from build123d import *

# Parameters (mm, degrees)
F0_R     = 1.95
F1_DEPTH = 30
F2_SIZE  = 1
F0_W     = 62.6598149538
F0_H     = 31.0992728919
F0_R_2   = 15
F3_DEPTH = 3
F4_D     = 3.3
F4_DEPTH = 10
F4_TIP   = 0.9914200214


with BuildPart() as f1:
    # F0 (on Top) → F1 (new body)
    with BuildSketch(Plane.XY):
        Circle(F0_R)
    extrude(amount=F1_DEPTH)

    # F2
    f2_edges = [f1.edges().sort_by_distance(p)[0] for p in [
        (-1.95, 0, 30),
    ]]
    chamfer(f2_edges, length=F2_SIZE)

    # F0 (on Top) → F3 (join)
    with BuildSketch(Plane.XY):
        Rectangle(F0_W, F0_H)
        Circle(F0_R_2, mode=Mode.SUBTRACT)
        Circle(F0_R_2)
        Circle(F0_R, mode=Mode.SUBTRACT)
        Circle(F0_R)
    extrude(amount=-F3_DEPTH)

    # F4
    with Locations(Plane.XY):
        with Locations((-26.3299074769, 10.5496364459), (26.3299074769, 10.5496364459), (26.3299074769, -10.5496364459), (-26.3299074769, -10.5496364459)):
            Hole(F4_D / 2, depth=F4_DEPTH)
            with Locations((0, 0, -(F4_DEPTH + F4_TIP / 2))):  # 118° drill point
                Cone(0, F4_D / 2, F4_TIP, mode=Mode.SUBTRACT)


solid = f1.part
Input: part model. Units: mm. Frame: model coordinates. Give positions to 0.01 mm unless a question says otherwise; leave off trailing zeros. Write each loop counter-clockwise with the first axis right and the second up, starting at its lowest first coordinate (ties: lowest second). Pieces come first, ordered by that corner, then holes.
Q1. First-contact query: P1, Ø3, axis at x = 5, z = 15.5, coming from the -Y side; P2, Ø8, axis at x = 4, y = -4, coming from the +Z side; P3, Ø4.5, axis at x = -26.33, y = 10.55, coming from the +Z side. Flat tips, straight axial feed; report the tip coordinate or a pass-through.
Q2. Section D-D, the plane x = 20. Output: boundary loops of the cut face in (y, z), plus the area to 3 significant figures.
Q3. Section C-C, the plane z = 12.5. Output: boundary loops of the cut face in (x, y).
Q4. Pull-direction query (Y, two-part tool) for faces 1 (the face through (-25.021, 9.546, -1.521)), 2 (the face through (-31.33, 0, -1)), 3 (the face through (-1.437, 1.318, 14.297)); classes: pulls with the +Y half, pulls with the -Y half, needs draft (parallel to the pull), parting line crosses it, or undercut.
Q5. Material intervals for probe 1 along Z at (x, y) = (21, 14); probe 2 along Y at (x, z) = (0.5, 17.5), sorted ascending.
Q6. Section A-A, the plane x = 0. Output: boundary loops of the cut face in (y, z).
Q7. Section B-B, the plane y = 0. Output: boundary loops of the cut face in (x, z), plus the area to 3 significant figures.
Filled in:
1. P1: passes through
1. P2: stops at z = 29.29
1. P3: stops at z = 0
2. outline: (-15.55, -3) - (15.55, -3) - (15.55, 0) - (-15.55, 0) - close
2. area: 93.3 mm2
3. outline: circle Ø3.9 at (0, 0)
4. face 1: undercut
4. face 2: needs draft
4. face 3: parting line crosses it
5. probe 1: z = -3 to 0
5. probe 2: y = -1.88 to 1.88
6. outline: (-15.55, -3) - (15.55, -3) - (15.55, 0) - (1.95, 0) - (1.95, 29) - (0.95, 30) - (-0.95, 30) - (-1.95, 29) - (-1.95, 0) - (-15.55, 0) - close
7. outline: (-31.33, -3) - (31.33, -3) - (31.33, 0) - (1.95, 0) - (1.95, 29) - (0.95, 30) - (-0.95, 30) - (-1.95, 29) - (-1.95, 0) - (-31.33, 0) - close
7. area: 304 mm2
